```python
from build123d import *

# Parameters (mm, degrees)
BOSS_EXTRUDE3_DEPTH = 11.557
SKETCH3_W           = 11.049
SKETCH3_H           = 26.9875
BOSS_EXTRUDE4_DEPTH = 1.5875
CUT_EXTRUDE1_REACH  = 28.988
SKETCH4_W           = 13.208
SKETCH4_H           = 7.874


with BuildPart() as part:
    # Sketch1 → Boss-Extrude3 (new body, symmetric)
    with BuildSketch(Plane(origin=(0, 0, 0), x_dir=(0, 0, -1), z_dir=(1, 0, 0))):
        Polygon((-5.5245, -13.49375), (-3.937, -13.49375), (-3.937, 11.90625), (3.937, 11.90625), (3.937, 3.65125), (0.508, 3.65125), (0.508, -11.58875), (-1.651, -11.58875), (-1.651, -13.49375), (5.5245, -13.49375), (5.5245, 13.49375), (-5.5245, 13.49375), align=None)
    extrude(amount=BOSS_EXTRUDE3_DEPTH, both=True)

    # Sketch3 → Boss-Extrude4 (add)
    with BuildSketch(Plane(origin=(11.557, 0, 0), x_dir=(0, 0, -1), z_dir=(1, 0, 0))):
        Rectangle(SKETCH3_W, SKETCH3_H)
    extrude(amount=BOSS_EXTRUDE4_DEPTH)

    # Sketch4 → Cut-Extrude1 (cut, up to next)
    with BuildSketch(Plane(origin=(0, 13.49375, 0), x_dir=(1, 0, 0), z_dir=(0, 1, 0)), mode=Mode.PRIVATE) as cut_extrude1_sk1:
        with Locations((-4.953, 0)):
            Rectangle(SKETCH4_W, SKETCH4_H)
    cut_extrude1_tool1 = extrude(cut_extrude1_sk1.sketch, amount=-CUT_EXTRUDE1_REACH, mode=Mode.PRIVATE) & part.part
    add(cut_extrude1_tool1.solids().sort_by_distance((-4.953, 13.49375, 0))[0], mode=Mode.SUBTRACT)


solid = part.part
```
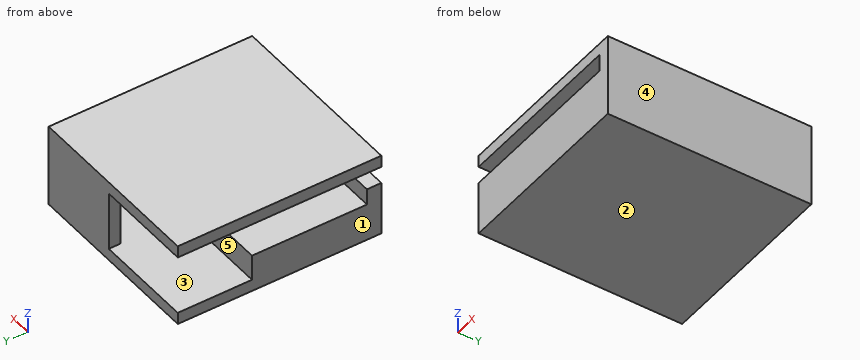
Design review of the part built by this model. Coordinates are the model's own, in mm. Face numbers are marked on the shaded views. A direction names the side the tool comes from. Round coordinates to 2 decimals unless told otherwise and drop trailing zeros. Write each loop counter-clockwise with the first axis right and the second up, starting at its lowest first coordinate (ties: lowest second). Pieces come first, ordered by that corner, then holes. Notation, with made-up numbers: (-8.5, 7.25) -> (50.5, 7.25) arc R22 cw to (50.5, 16.25) -> close; hole circle Ø11 at (-19, 65). An arc over 180 degrees is marked (long way). Answer in a Markdown table with one row per item.
Q1. Take a section at A-A, the plane y = -1.5. State the section outline as (x, z) points.
The answers:
| item | result |
|---|---|
| outline | (-11.56, -5.52) -> (13.14, -5.52) -> (13.14, 5.52) -> (-11.56, 5.52) -> (-11.56, 3.94) -> (11.56, 3.94) -> (11.56, -0.51) -> (-11.56, -0.51) -> close |
Q2. To check wall thickness, follow L1, parallel to Z at x = 5.75, y = -1; L2, parallel to Z at x = 10, y = 11; L3, parallel to Y at x = 7.25, z = -1. State the ranges of each line that lie inside material, in increasing order. Write a range as [from, to].
The answers:
| item | result |
|---|---|
| L1 | [-5.52, -0.51], [3.94, 5.52] |
| L2 | [-5.52, -3.94], [3.94, 5.52] |
| L3 | [-13.49, 3.65], [11.91, 13.49] |
Q3. For the marked faces 4 and 5, list the 3-axis set-ups (+Z, -Z, +X, -X, +Y, -Y) from which the entire face can be reached by the end or side of a thin tool; tool diameter is ignored.
The answers:
| item | result |
|---|---|
| face 4 | +Z, -Z, +X, +Y, -Y |
| face 5 | -X |
Q4. Take a section at D-D, the plane z = -1.75. State the section outline as (x, y) points, then the cut area to 3 significant figures.
The answers:
| item | result |
|---|---|
| outline | (-11.56, -13.49) -> (13.14, -13.49) -> (13.14, 13.49) -> (1.65, 13.49) -> (1.65, 11.91) -> (11.56, 11.91) -> (11.56, 3.65) -> (-11.56, 3.65) -> close |
| area | 455 mm² |
Q5. Take a section at C-C, the plane x = -0.75. State the section outline as (y, z) points.
The answers:
| item | result |
|---|---|
| outline | (-13.49, -5.52) -> (13.49, -5.52) -> (13.49, -3.94) -> (3.65, -3.94) -> (3.65, -0.51) -> (-11.59, -0.51) -> (-11.59, 1.65) -> (-13.49, 1.65) -> close; (-13.49, 3.94) -> (13.49, 3.94) -> (13.49, 5.52) -> (-13.49, 5.52) -> close |
Q6. Draft analysis for pull direction Z (two halves, no side actions). For the marked faces 1, 2 and 3, state which applies: +Z half, -Z half, draft (parallel to the pull), parting line (faces both ways), or undercut.
The answers:
| item | result |
|---|---|
| face 1 | draft |
| face 2 | -Z half |
| face 3 | undercut |
Q7. Take a section at B-B, the plane x = 9. State the section outline as (y, z) points, then the cut area to 3 significant figures.
The answers:
| item | result |
|---|---|
| outline | (-13.49, -5.52) -> (13.49, -5.52) -> (13.49, 5.52) -> (-13.49, 5.52) -> (-13.49, 3.94) -> (11.91, 3.94) -> (11.91, -3.94) -> (3.65, -3.94) -> (3.65, -0.51) -> (-11.59, -0.51) -> (-11.59, 1.65) -> (-13.49, 1.65) -> close |
| area | 161 mm² |
Q8. Clearance check with flat-ended pins moving along their axes: pin 1 Ø2.5 at (x, z) = (-4, 0.5) entering from +Y; pin 2 Ø1.7 at (y, z) = (12.5, 2) entering from -X. State where each tip first meets the part, or that it passes through.
The answers:
| item | result |
|---|---|
| pin 1 | y = 3.65 |
| pin 2 | x = 1.65 |
